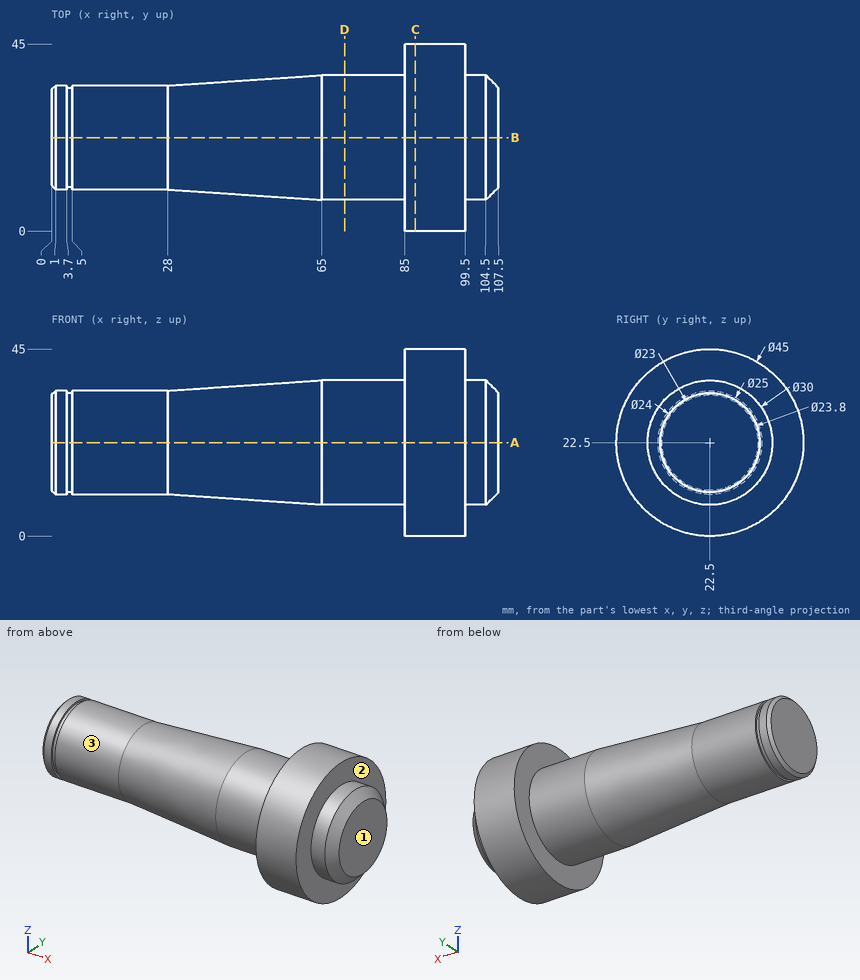
The figure shows three views and two pictorial views of one solid part (mm, origin at its lowest corner). Answer the questions. A direction names the side the tool comes from. Coordinates: 2 decimals unless noted, no trailing zeros. Write each loop counter-clockwise with the first axis right and the second up, starting at its lowest first coordinate (ties: lowest second). Pieces come first, ordered by that corner, then holes. Notation, with made-up numbers: (6.25, -25.5) -> (48.25, -25.5) arc R4 cw to (48.25, -21.5) -> close; hole circle Ø9 at (-28.75, 53). An arc over 180 degrees is marked (long way). Return JSON: item names as keys, results as strings.
(1) Consider line 1 along Y through (x, z) = (71.5, 13.5); line 2 along X through (y, z) = (27, 41); line 3 along X through (y, z) = (33, 16). Determine where each line is inside the solid, lowest interval first. Write a range as from..to.
Answers below:
{"line 1": "10.5..34.5", "line 2": "85..99.5", "line 3": "0.85..3.7, 5..107.15"}
(2) Each of these flat-tipped pins is pushed along its axis until it touches: P1, Ø3, axis at y = 9, z = 11, coming from the -X side; P2, Ø3, axis at x = 92.5, y = 17, coming from the -Z side; P3, Ø4, axis at x = 92.5, z = 15.5, coming from the -Y side. Where does it stop, or does it pass through?
Answers below:
{"P1": "x = 85", "P2": "z = 0.36", "P3": "y = 0.56"}
(3) Which of the six approach directions +Z, -Z, +X, -X, +Y, -Y give full straight-line access (tool end or side, diameter ignored) to the marked faces 1, 2 and 3?
Answers below:
{"face 1": "+Z, -Z, +X, +Y, -Y", "face 2": "+X", "face 3": "-X"}
(4) The part is cut by section D-D on x = 70.5. Give the vertices of the cut face in (y, z).
Answers below:
{"outline": "circle Ø30 at (22.5, 22.5)"}
(5) The part is cut by section C-C on x = 87.5. Give the vertices of the cut face in (y, z).
Answers below:
{"outline": "circle Ø45 at (22.5, 22.5)"}
(6) The part is cut by section A-A on z = 22.5. Give the vertices of the cut face in (x, y).
Answers below:
{"outline": "(0, 11) -> (1, 10) -> (3.7, 10) -> (3.7, 10.6) -> (5, 10.6) -> (5, 10) -> (28, 10) -> (65, 7.5) -> (85, 7.5) -> (85, 0) -> (99.5, 0) -> (99.5, 7.5) -> (104.5, 7.5) -> (107.5, 10.5) -> (107.5, 34.5) -> (104.5, 37.5) -> (99.5, 37.5) -> (99.5, 45) -> (85, 45) -> (85, 37.5) -> (65, 37.5) -> (28, 35) -> (5, 35) -> (5, 34.4) -> (3.7, 34.4) -> (3.7, 35) -> (1, 35) -> (0, 34) -> close"}
